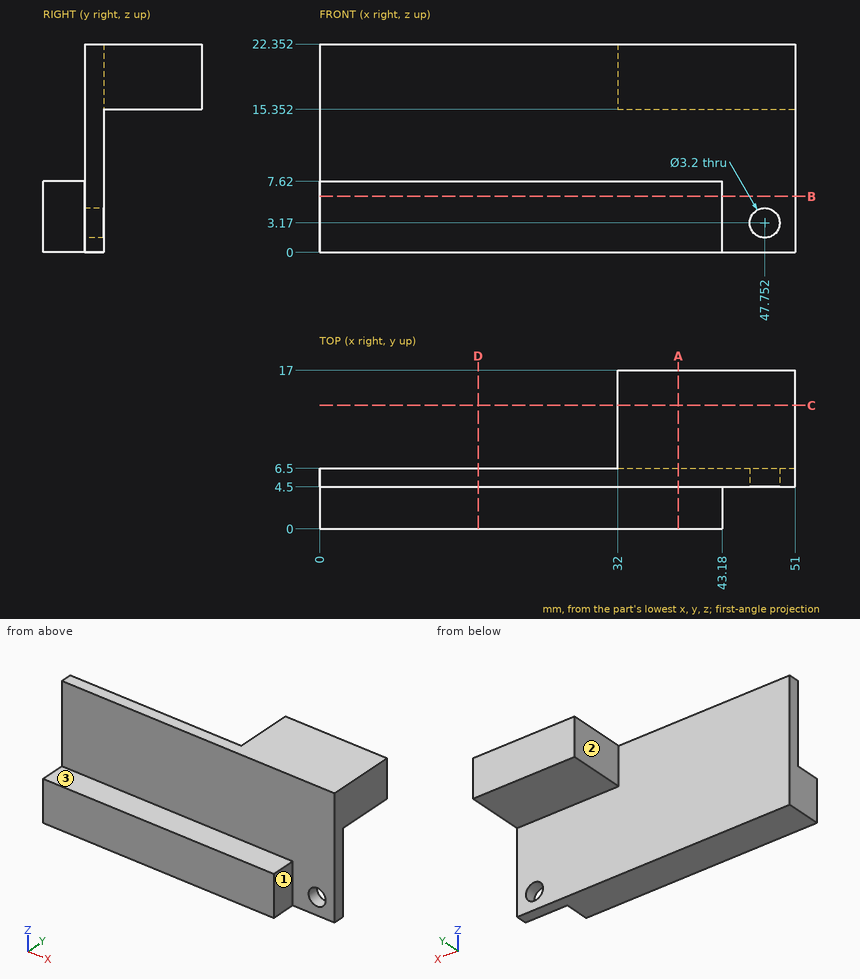
Check sheet for the drawn part. Datum: minimum x, y, z corner. Units: mm. A direction names the side the tool comes from. Give positions to 0.01 mm unless a question says otherwise; leave off trailing zeros. Write each loop counter-clockwise with the first axis right and the second up, starting at its lowest first coordinate (ties: lowest second). Pieces come first, ordered by that corner, then holes. Notation, with made-up numbers: M 50,23.5 L 109,23.5 A10 ccw 109,27.5 Z; hole C 20,-24 d2. An arc over 180 degrees is marked long. Write item = value, one per line.
(1) Material ranges on line 1 (Y direction, x = 36, z = 14); line 2 (Z direction, x = 48.5, y = 6.75); line 3 (Y direction, x = 10.5, z = 5.25), recorded low to high.
Found:
line_1 = 4.5 to 6.5
line_2 = 15.35 to 22.35
line_3 = 0 to 6.5
(2) Sectioned sample at C-C (y = 13.25). Record the cut outline in (x, z), then the cut area to 3 significant figures.
Found:
outline = M 32,15.35 L 51,15.35 L 51,22.35 L 32,22.35 Z
area = 133 mm2
(3) Go/stop test with flat-tipped pins: pin 1 Ø8 at (x, y) = (10, 14) entering from -Z; pin 2 Ø1.3 at (x, y) = (11.5, 2) entering from +Z; pin 3 Ø2 at (y, z) = (12, 18) entering from -X; pin 4 Ø5 at (x, y) = (45.5, 9.5) entering from -Z. Record where each tip stops, or that it passes through.
Found:
pin_1 = through
pin_2 = 7.62
pin_3 = 32
pin_4 = 15.35
(4) Access from +Z, -Z, +X, -X, +Y, -Y to the whole of each face (thin tool, end or side, straight path). Record for the marked faces 1, 2 and 3.
Found:
face_1 = +Z, -Z, +X, -Y
face_2 = +Z, -Z, -X, +Y
face_3 = +Z, +X, -X, -Y
(5) Sectioned sample at A-A (x = 38.5). Record the cut outline in (y, z).
Found:
outline = M 0,0 L 6.5,0 L 6.5,15.35 L 17,15.35 L 17,22.35 L 4.5,22.35 L 4.5,7.62 L 0,7.62 Z
(6) Sectioned sample at D-D (x = 17). Record the cut outline in (y, z).
Found:
outline = M 0,0 L 6.5,0 L 6.5,22.35 L 4.5,22.35 L 4.5,7.62 L 0,7.62 Z
(7) Sectioned sample at B-B (z = 6). Record the cut outline in (x, y).
Found:
outline = M 0,0 L 43.18,0 L 43.18,4.5 L 51,4.5 L 51,6.5 L 0,6.5 Z
